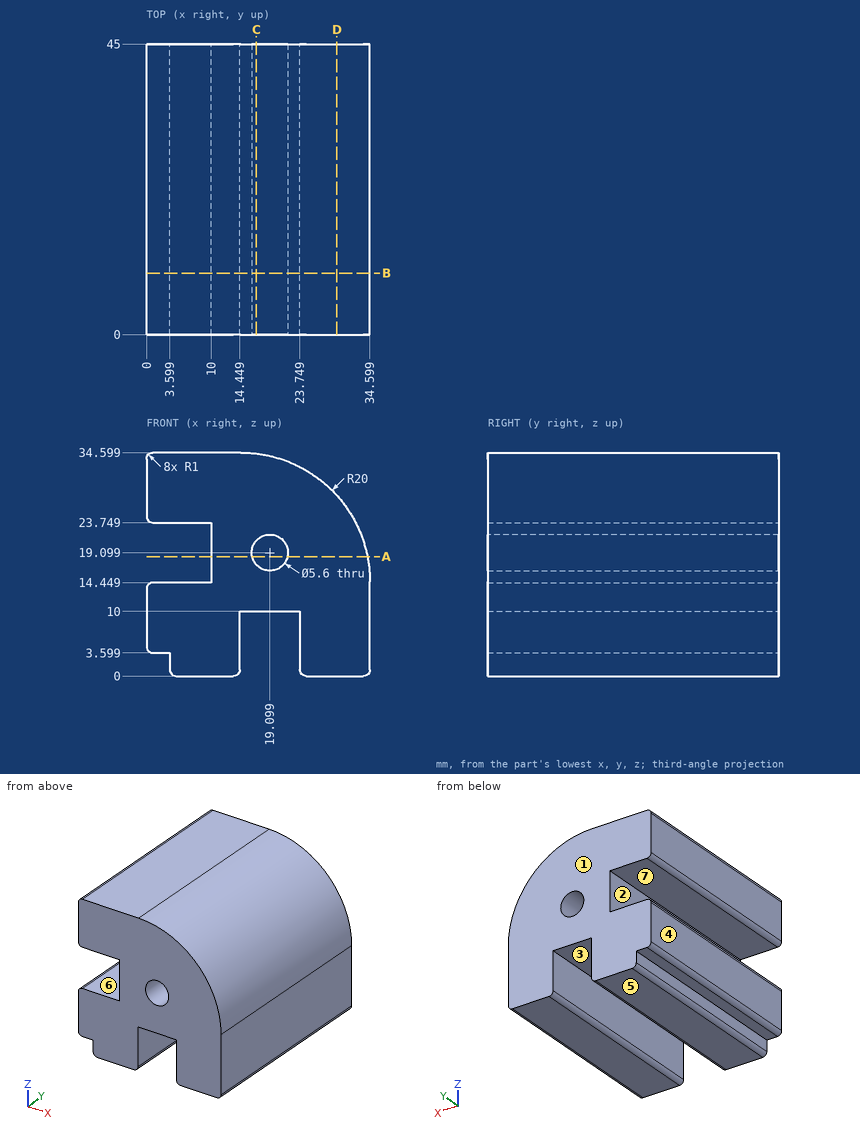
Source: three-view drawing plus pictorial views. Frame: mm from the lowest corner of the part. A direction names the side the tool comes from. Coordinates: 2 decimals unless noted, no trailing zeros. Loops run counter-clockwise (first coordinate to the right, second up) from the corner with the lowest first, then second, coordinate; pieces in that order, holes last. Notation, with made-up numbers: (26.5, -3.75) - (50.5, -3.75) arc R23 cw to (50.5, 23.25) - close; hole circle Ø4 at (77.5, 61). An arc over 180 degrees is marked (long way). One line per item, written item: value. Start each with the question number.
1. Ray query, L1, parallel to X at y = 14, z = 8.5; L2, parallel to Z at x = 31, y = 34 (1 decimal). Return the intervals inside material, ascending.
2. Contact query for flat-ended pins moving along their axis: P1, Ø2, axis at y = 16.5, z = 1.5, coming from the -X side; P2, Ø12, axis at x = 6, y = 24, coming from the -Z side; P3, Ø2, axis at x = 3, y = 12.5, coming from the -Z side; P4, Ø3, axis at x = 21, y = 28, coming from the -Z side. Output: stop coordinate, or through.
3. Section A-A (z = 18.5). Return the cut outline in (x, y) (1 decimal).
4. Section D-D (x = 29.5). Return the cut outline in (y, z).
5. Set-up query: the marked faces 1, 2 and 3. Return all of +Z, -Z, +X, -X, +Y, -Y with unobstructed straight access to the full face (end or side cutting, diameter ignored); none if empty.
6. Mould query, pull axis Z, two halves, no side actions, for the marked faces 4, 5, 6 and 7. Classes: pulls with the +Z half, pulls with the -Z half, needs draft (parallel to the pull), parting line crosses it, or undercut.
7. Section C-C (x = 17). Return the cut outline in (y, z), and give its area (3 significant figures).
8. Section B-B (y = 9.5). Return the cut outline in (x, z), and give its area (3 significant figures).
Verdict:
1. L1: x = 0 to 14.45, 23.75 to 34.6
1. L2: z = 0 to 26
2. P1: stops at x = 3.6
2. P2: stops at z = 0
2. P3: stops at z = 0.2
2. P4: stops at z = 10
3. outline: (10, 0) - (16.4, 0) - (16.4, 45) - (10, 45) - close; (21.8, 0) - (34.2, 0) - (34.2, 45) - (21.8, 45) - close
4. outline: (0, 0) - (45, 0) - (45, 27.94) - (0, 27.94) - close
5. face 1: +Z, -Z, +X, -X, +Y
5. face 2: -X, +Y, -Y
5. face 3: -Z, +Y, -Y
6. face 4: needs draft
6. face 5: pulls with the -Z half
6. face 6: undercut
6. face 7: undercut
7. outline: (0, 10) - (45, 10) - (45, 17.25) - (0, 17.25) - close; (0, 20.95) - (45, 20.95) - (45, 34.45) - (0, 34.45) - close
7. area: 934 mm2
8. outline: (0, 4.6) arc R1 ccw to (1, 3.6) - (3.6, 3.6) - (3.6, 1) arc R1 ccw to (4.6, 0) - (13.45, 0) arc R1 ccw to (14.45, 1) - (14.45, 10) - (23.75, 10) - (23.75, 1) arc R1 ccw to (24.75, 0) - (33.6, 0) arc R1 ccw to (34.6, 1) - (34.6, 14.6) arc R20 ccw to (14.6, 34.6) - (1, 34.6) arc R1 ccw to (0, 33.6) - (0, 24.75) arc R1 ccw to (1, 23.75) - (10, 23.75) - (10, 14.45) - (1, 14.45) arc R1 ccw to (0, 13.45) - close; hole circle Ø5.6 at (19.1, 19.1)
8. area: 886 mm2
